Here's how the part is built. I have some questions about the finished solid (model axes, mm). Face numbers are marked on the shaded views. A direction names the side the tool comes from. Coordinates: 2 decimals unless noted, no trailing zeros. Loops run counter-clockwise (first coordinate to the right, second up) from the corner with the lowest first, then second, coordinate; pieces in that order, holes last. Notation, with made-up numbers: (8.25, -22.5) -> (63.25, -22.5) arc R27 cw to (63.25, 9.5) -> close; hole circle Ø8 at (-21.5, 70.5). An arc over 180 degrees is marked (long way). Answer as a JSON object with one key per item and string values. Group by question number.
1) I want a section at D-D (y = -6.25). Write out the boundary of the cut face in (x, z).
2) I want a section at B-B (y = 13.5). Write out the boundary of the cut face in (x, z).
3) I want a section at C-C (z = 9.5). Write out the boundary of the cut face in (x, y), then the cut area to 3 significant figures.
4) I need wall thicknesses on probe 1 along X at (y, z) = (-0.5, 1.25); probe 2 along Z at (x, y) = (4, 15); probe 3 along X at (y, z) = (-8, 6.5). Which ranges of each line are inside material? Lowest first, please. Write a range as [from, to].
5) Which directions (+Z, -Z, +X, -X, +Y, -Y) give clear straight access to the entire face, cutting with the end or side of a thin tool? Please do the marked faces 3 and 4.
6) I'm going to push flat-ended pins straight in: pin 1 (6 mm diameter, centred on x = -14.5, z = 1.5, fed in from +Y); pin 2 (4 mm diameter, centred on y = 15, z = 6.5, fed in from -X); pin 3 (1 mm diameter, centred on x = 3.5, y = -9, fed in from +Z). Where does each tip first touch, or does it pass through?
7) I want a section at A-A (x = 0). Write out the boundary of the cut face in (y, z), then the cut area to 3 significant figures.
8) If we mould it in two halves opening along Y, with no side actions, what happens to the marked faces 1 and 2? For each: +Y half, -Y half, draft (parallel to the pull), parting line (faces both ways), or undercut.
```python
from build123d import *

# Parameters (mm, degrees)
F0_R            = 19.5
F0_R_2          = 2.1
F1_DEPTH        = 2
F2_DEPTH        = 10
F2_COPIES_COUNT = 3


# Not quite as in the source:
# - a pattern or mirror of a feature is missing from the dataset's text; its kind, count and spacing are read off the source's solid


with BuildPart() as f1:
    # F0 (on Top) → F1 (new body)
    with BuildSketch(Plane.XY):
        Circle(F0_R)
        with Locations((9.1651513899, 8.5)):
            Circle(F0_R_2, mode=Mode.SUBTRACT)
        with Locations((0, 12.5)):
            Circle(F0_R_2, mode=Mode.SUBTRACT)
    extrude(amount=F1_DEPTH)

    # F0 (on Top) → F2 (join)
    with BuildSketch(Plane.XY):
        with Locations((0, 12.5)):
            Circle(F0_R_2)
        with Locations((9.1651513899, 8.5)):
            Circle(F0_R_2)
    f2 = extrude(amount=F2_DEPTH)

    # F2_copies: F2 ×3 about axis
    f2_copies_axis = Axis((0, 0, 0), (0, 0, 1))
    for i in range(1, F2_COPIES_COUNT):
        add(f2.rotate(f2_copies_axis, i * 360 / F2_COPIES_COUNT))


solid = f1.part
```
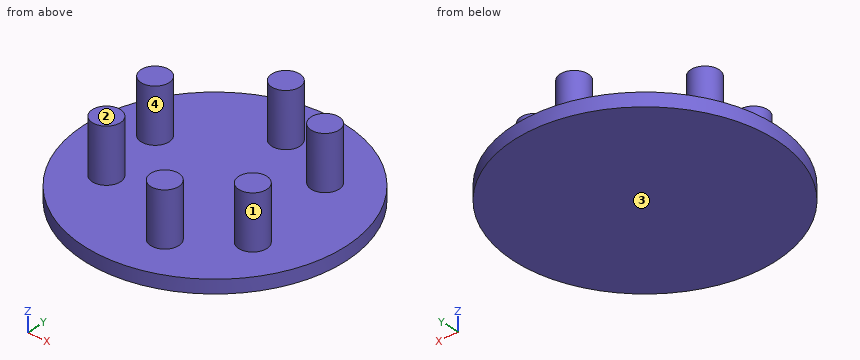
Determined:
{
 "1": {"outline": "(-18.47, 0) -> (18.47, 0) -> (18.47, 2) -> (12.93, 2) -> (12.93, 10) -> (8.73, 10) -> (8.73, 2) -> (-8.73, 2) -> (-8.73, 10) -> (-12.93, 10) -> (-12.93, 2) -> (-18.47, 2) -> close"},
 "2": {"outline": "(-14.07, 0) -> (14.07, 0) -> (14.07, 2) -> (1.85, 2) -> (1.85, 10) -> (-1.85, 10) -> (-1.85, 2) -> (-14.07, 2) -> close"},
 "3": {"outline": "circle Ø4.2 at (-11.94, 3.69); circle Ø4.2 at (-10.83, -6.25); circle Ø4.2 at (0, 12.5); circle Ø4.2 at (2.78, -12.19); circle Ø4.2 at (9.17, 8.5); circle Ø4.2 at (10.83, -6.25)", "area": "83.1 mm^2"},
 "4": {"probe 1": "[-19.49, 19.49]", "probe 2": "[0, 2]", "probe 3": "[-11.99, -9.66], [9.66, 11.99]"},
 "5": {"face 3": "-Z, +X, -X, +Y, -Y", "face 4": "+Z"},
 "6": {"pin 1": "y = 15.75", "pin 2": "x = -2.04", "pin 3": "z = 2"},
 "7": {"outline": "(-19.5, 0) -> (19.5, 0) -> (19.5, 2) -> (14.6, 2) -> (14.6, 10) -> (10.4, 10) -> (10.4, 2) -> (-19.5, 2) -> close", "area": "112 mm^2"},
 "8": {"face 1": "undercut", "face 2": "draft"}
}
